from build123d import *

# Parameters (mm, degrees)
F1_DEPTH = 30
F2_R     = 4.4
F3_R     = 4.4
F4_DEPTH = 25
F5_R     = 2
F6_R     = 2


# Not quite as in the source:
# - a feature names something its author has since deleted; it is built from what else it names


with BuildPart() as f1:
    # F0 (on Front) → F1 (new body)
    with BuildSketch(Plane.XZ):
        Polygon((90, -1), (90, 1), (70, 1), (70, 54), (-70, 54), (-70, 1), (-90, 1), (-90, -1), (-68, -1), (-68, 52), (68, 52), (68, -1), align=None)
    extrude(amount=F1_DEPTH)

    # F2 (on face) + F3 (on face) → F4 (cut)
    with BuildSketch(Plane.XY.offset(1)):
        with Locations((-80, -15)):
            Circle(F2_R)
        with Locations((80, -15)):
            Circle(F2_R)
    with BuildSketch(Plane.XY.offset(54)):
        with Locations((-25, -15)):
            Circle(F3_R)
        with Locations((25, -15)):
            Circle(F3_R)
    extrude(amount=-F4_DEPTH, mode=Mode.SUBTRACT)

    # F5
    f5_edges = [f1.edges().sort_by_distance(p)[0] for p in [
        (-70, -15, 54),
        (70, -15, 54),
    ]]
    fillet(f5_edges, radius=F5_R)

    # F6
    f6_edges = [f1.edges().sort_by_distance(p)[0] for p in [
        (68, -15, -1),
        (-68, -15, -1),
    ]]
    fillet(f6_edges, radius=F6_R)


solid = f1.part
Design review of the part built by this model. Coordinates are the model's own, in mm. A direction names the side the tool comes from. Give positions to 0.01 mm unless a question says otherwise; leave off trailing zeros. Write each loop counter-clockwise with the first axis right and the second up, starting at its lowest first coordinate (ties: lowest second). Pieces come first, ordered by that corner, then holes. Notation, with made-up numbers: M -38,75 L 9,75 A20 cw 9,89 Z; hole C -35,-33.75 d6. An arc over 180 degrees is marked long. Return JSON: item names as keys, results as strings. Group by question number.
Item 1: Take a section at C-C (y = -15). Count the separate pieces of the cut face and the enclosed holes in it, plus the area to 3 significant figures.
Item 2: Take a section at D-D (y = -7.75). Give the boundary of the cut face in (x, z), plus the area to 3 significant figures.
Item 3: Take a section at B-B (z = 10). Give the boundary of the cut face in (x, y).
Item 4: Clearance check with flat-ended pins moving along their axes: pin 1 Ø7 at (x, y) = (-25, -15) entering from +Z; pin 2 Ø11.5 at (x, y) = (-80, -15) entering from +Z; pin 3 Ø9 at (y, z) = (-22, 16) entering from -X; pin 4 Ø10 at (x, y) = (25, -15) entering from -Z. State where each tip first meets the part, or that it passes through.
Item 5: Tool access review of faces 1 (the flat face through (85, -15, 1)), 2 (the flat face through (-85, -15, -1)), 3 (the flat face through (-70, -15, 27)), 4 (the flat face through (-68, -15, 26)): name each direction out of +Z, -Z, +X, -X, +Y, -Y from which nothing blocks a thin tool from reaching the whole face with its end or side.
Item 6: The part is to be moulded in two halves that separate along X. For faces 5 (the cylindrical face through (75.604, -14.807, 0.014)), 6 (the flat face through (0, 0, 53)), 7 (the flat face through (68, -15, 27)), 8 (the flat face through (70, -15, 26)), say which applies: pulls with the +X half, pulls with the -X half, needs draft (parallel to the pull), parting line crosses it, or undercut.
Item 7: Take a section at A-A (x = 80). Give the boundary of the cut face in (y, z), plus the area to 3 significant figures.
Item 8: Wall thickness on line 1 along X through (y, z) = (-18, 27.5); line 2 along Y through (x, z) = (-80, 0.4); line 3 along Z through (x, y) = (-20.5, -2.5): over which ranges is each line inside the solid? List them lowest first.
Return value:
{
 "1": {"separate pieces": "5", "enclosed holes": "0", "area": "498 mm2"},
 "2": {"outline": "M -90,-1 L -70,-1 A2 ccw -68,1 L -68,52 L 68,52 L 68,1 A2 ccw 70,-1 L 90,-1 L 90,1 L 70,1 L 70,52 A2 ccw 68,54 L -68,54 A2 ccw -70,52 L -70,1 L -90,1 Z", "area": "569 mm2"},
 "3": {"outline": "M -70,-30 L -68,-30 L -68,0 L -70,0 Z; M 68,-30 L 70,-30 L 70,0 L 68,0 Z"},
 "4": {"pin 1": "passes through", "pin 2": "stops at z = 1", "pin 3": "stops at x = -70", "pin 4": "stops at z = 52"},
 "5": {"face 1": "+Z, +X, +Y, -Y", "face 2": "-Z, +X, -X, +Y, -Y", "face 3": "+Z, -X, +Y, -Y", "face 4": "-Z, +Y, -Y"},
 "6": {"face 5": "undercut", "face 6": "needs draft", "face 7": "undercut", "face 8": "pulls with the +X half"},
 "7": {"outline": "M -30,-1 L -19.4,-1 L -19.4,1 L -30,1 Z; M -10.6,-1 L 0,-1 L 0,1 L -10.6,1 Z", "area": "42.4 mm2"},
 "8": {"line 1": "x = -70 to -68, 68 to 70", "line 2": "y = -30 to -19.4, -10.6 to 0", "line 3": "z = 52 to 54"}
}
